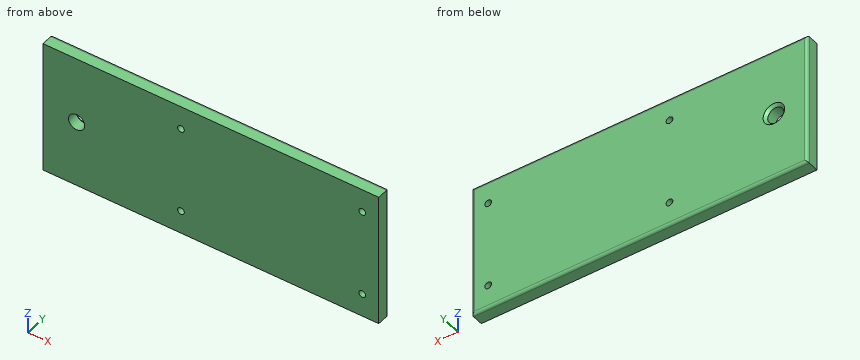
```python
from build123d import *

# Parameters (mm, degrees)
SKETCH1_W           = 250
SKETCH1_H           = 100
BOSS_EXTRUDE1_DEPTH = 10
FILLET1_R           = 2
SKETCH2_R           = 6
CUT_EXTRUDE1_DEPTH  = 11
CHAMFER1_SIZE       = 2
SKETCH3_R           = 2.5
CUT_EXTRUDE2_DEPTH  = 11


with BuildPart() as part:
    # Sketch1 → Boss-Extrude1 (new body)
    with BuildSketch(Plane(origin=(0, 0, 0), x_dir=(1, 0, 0), z_dir=(0, 1, 0))):
        Rectangle(SKETCH1_W, SKETCH1_H)
    extrude(amount=BOSS_EXTRUDE1_DEPTH)

    # Fillet1
    fillet1_edges = [part.edges().sort_by_distance(p)[0] for p in [
        (125, 10, 0),
        (0, 10, -50),
        (-125, 10, 0),
        (0, 10, 50),
    ]]
    fillet(fillet1_edges, radius=FILLET1_R)

    # Sketch2 → Cut-Extrude1 (cut, through all)
    with BuildSketch(Plane(origin=(0, 10, 0), x_dir=(1, 0, 0), z_dir=(0, 1, 0))):
        with Locations((-100, 0)):
            Circle(SKETCH2_R)
    extrude(amount=-CUT_EXTRUDE1_DEPTH, mode=Mode.SUBTRACT)

    # Chamfer1
    chamfer1_edges = [part.edges().sort_by_distance(p)[0] for p in [
        (-106, 10, 0),
    ]]
    chamfer(chamfer1_edges, length=CHAMFER1_SIZE)

    # Sketch3 → Cut-Extrude2 (cut, through all)
    with BuildSketch(Plane(origin=(0, 10, 0), x_dir=(1, 0, 0), z_dir=(0, 1, 0))):
        with Locations((112.723846374, 32.5)):
            Circle(SKETCH3_R)
        with Locations((112.723846374, -32.5)):
            Circle(SKETCH3_R)
        with Locations((-22.276153626, 32.5)):
            Circle(SKETCH3_R)
        with Locations((-22.276153626, -32.5)):
            Circle(SKETCH3_R)
    extrude(amount=-CUT_EXTRUDE2_DEPTH, mode=Mode.SUBTRACT)


solid = part.part
```
The model under review builds one solid part; all positions refer to its coordinate system, in mm. Coordinates: 2 decimals unless noted, no trailing zeros. Write each loop counter-clockwise with the first axis right and the second up, starting at its lowest first coordinate (ties: lowest second). Pieces come first, ordered by that corner, then holes.
1) We need section C-C on z = -32.5. State the section outline as (x, y) points.
2) To check wall thickness, follow probe 1 along X at (y, z) = (3, -32.5); probe 2 along Z at (x, y) = (-100, 2.5); probe 3 along Z at (x, y) = (-98, 9.25). State the ranges of each line that lie inside material, in increasing order.
3) We need section A-A on x = -100. State the section outline as (y, z) points.
4) We need section B-B on z = 0. State the section outline as (x, y) points.
Answer list:
1. outline: (-125, 0) - (-24.78, 0) - (-24.78, 10) - (-123, 10) arc R2 ccw to (-125, 8) - close; (-19.78, 0) - (110.22, 0) - (110.22, 10) - (-19.78, 10) - close; (115.22, 0) - (125, 0) - (125, 8) arc R2 ccw to (123, 10) - (115.22, 10) - close
2. probe 1: x = -125 to -24.78, -19.78 to 110.22, 115.22 to 125
2. probe 2: z = -50 to -6, 6 to 50
2. probe 3: z = -49.56 to -6.97, 6.97 to 49.56
3. outline: (0, -50) - (8, -50) arc R2 ccw to (10, -48) - (10, -8) - (8, -6) - (0, -6) - close; (0, 6) - (8, 6) - (10, 8) - (10, 48) arc R2 ccw to (8, 50) - (0, 50) - close
4. outline: (-125, 0) - (-106, 0) - (-106, 8) - (-108, 10) - (-123, 10) arc R2 ccw to (-125, 8) - close; (-94, 0) - (125, 0) - (125, 8) arc R2 ccw to (123, 10) - (-92, 10) - (-94, 8) - close
